Work out the finished part from the listing and answer in its coordinate system (mm). A direction names the side the tool comes from. Coordinates: 2 decimals unless noted, no trailing zeros. Write each loop counter-clockwise with the first axis right and the second up, starting at its lowest first coordinate (ties: lowest second). Pieces come first, ordered by that corner, then holes. Notation, with made-up numbers: (69, -2.75) - (87, -2.75) arc R21 cw to (87, 21.25) - close; hole circle Ø3 at (52.5, 12). An arc over 180 degrees is marked (long way). Use CSV: the item, a comma, the result in double quotes. Start each with the question number.
from build123d import *

# Parameters (mm, degrees)
F1_DEPTH = 6.35
F3_DEPTH = 52.578
F4_DEPTH = 45.974
F6_DEPTH = 4.064
F7_DEPTH = 3.81
F8_R     = 5.2545700387
F9_DEPTH = 25.4


with BuildPart() as f1:
    # F0 (on Front) → F1 (new body)
    with BuildSketch(Plane.XZ):
        Polygon((-31.1878696084, 40.077868849), (-52.4655729532, 40.077868849), (-52.4655729532, -4.226393532), (30.0219655037, -4.226393532), (30.0219655037, 19.6718552087), align=None)
    extrude(amount=F1_DEPTH)

    # F2 (on Right) → F3 (join)
    with BuildSketch(Plane.YZ):
        Polygon((-6.1209839769, -4.226393532), (-6.7039346322, 32.7909812331), (-16.3226239383, 32.7909812331), (-25.3583602607, 8.5985241458), (-25.3583602607, -4.226393532), align=None)
    extrude(amount=-F3_DEPTH)

    # F4 (cut): a face of the model
    f4_faces = [f1.faces().sort_by_distance(p)[0] for p in [
        (0, -14.7154551351, 12.274399221),
    ]]
    extrude(f4_faces, amount=-F4_DEPTH, mode=Mode.SUBTRACT)

    # F5 (on Top) → F6 (join)
    with BuildSketch(Plane.XY):
        Polygon((-46.0531152785, -6.2667215243), (-46.0531152785, -25.212623179), (-14.5737715065, -6.2667215243), align=None)
    extrude(amount=-F6_DEPTH)

    # F7 (add): a face of the model
    f7_faces = [f1.faces().sort_by_distance(p)[0] for p in [
        (-35.5533806316, -12.6216691671, 0),
    ]]
    extrude(f7_faces, amount=F7_DEPTH)

    # F8 (on face) → F9 (cut)
    with BuildSketch(Plane.XZ.offset(6.35)):
        with Locations((18.0714763701, 7.7227308384)):
            Circle(F8_R)
    extrude(amount=-F9_DEPTH, mode=Mode.SUBTRACT)


solid = f1.part
Item 1: Determine the mould class of faces 1 (the face through (-0.15, -3.13, 29.73)), 2 (the face through (-34, -14, -4.064)), 3 (the face through (22.925, -3.219, 5.71)) for opening direction X: +X half, -X half, draft (parallel to the pull), parting line (faces both ways), or undercut.
Item 2: A cutting plane is placed at D-D (z = 1). Determine the outline of the cut face in (x, y) (3 decimals), then the cut area to 3 significant figures.
Item 3: A cutting plane is placed at C-C (x = -40.5). Determine the outline of the cut face in (y, z), then the cut area to 3 significant figures.
Item 4: Straight lines are drawn through the part: probe 1 along Z at (x, y) = (-31, -11.75); probe 2 along X at (y, z) = (-9.25, 5); probe 3 along X at (y, z) = (-1.5, 15). For each, find the intervals that lie inside material, in ascending order. Write a range as [from, to].
Item 5: A cutting plane is placed at A-A (z = 26). Determine the outline of the cut face in (x, y), then the cut area to 3 significant figures.
Item 6: A cutting plane is placed at B-B (y = -17.75). Determine the outline of the cut face in (x, z), then the cut area to 3 significant figures.
Item 7: Which of the six approach directions +Z, -Z, +X, -X, +Y, -Y give full straight-line access (tool end or side, diameter ignored) to faces 4 (the face through (-34, -14, 3.81)), 5 (the face through (-18, -6, -4.226)), 6 (the face through (-49, -11, 32.791))?
Item 8: Each of these flat-tipped pins is pushed along its axis until it touches: pin 1 (5 mm diameter, centred on x = -38, z = 19.5, fed in from -Y); pin 2 (2 mm diameter, centred on x = -49, y = -10, fed in from +Z); pin 3 (1.5 mm diameter, centred on x = 14, z = 7.5, fed in from +Y); pin 4 (1.9 mm diameter, centred on y = -3.5, z = 12.5, fed in from -X). Where does it stop, or does it pass through?
Calculated:
1,face 1,"+X half"
1,face 2,"draft"
1,face 3,"undercut"
2,outline,"(-52.578, -25.358) - (-45.974, -25.358) - (-45.974, -25.165) - (-14.712, -6.35) - (30.022, -6.35) - (30.022, 0) - (-52.466, 0) - (-52.466, -6.203) - (-52.578, -6.203) - close"
2,area,"943 mm²"
3,outline,"(-21.87, -4.06) - (-6.35, -4.06) - (-6.35, -4.23) - (0, -4.23) - (0, 40.08) - (-6.35, 40.08) - (-6.35, 3.81) - (-21.87, 3.81) - close"
3,area,"404 mm²"
4,probe 1,"z = [-4.06, 3.81]"
4,probe 2,"x = [-52.58, -45.97]"
4,probe 3,"x = [-52.47, 30.02]"
5,outline,"(-52.58, -18.86) - (-45.97, -18.86) - (-45.97, -6.6) - (-52.58, -6.6) - close; (-52.47, -6.35) - (11.04, -6.35) - (11.04, 0) - (-52.47, 0) - close"
5,area,"484 mm²"
6,outline,"(-52.58, -4.23) - (-45.97, -4.23) - (-45.97, -4.06) - (-33.65, -4.06) - (-33.65, 3.81) - (-45.97, 3.81) - (-45.97, 28.97) - (-52.58, 28.97) - close"
6,area,"316 mm²"
7,face 4,"+Z, +X, -Y"
7,face 5,"-Z, +X, -X, +Y, -Y"
7,face 6,"+Z, +X, -X, -Y"
8,pin 1,"stops at y = -6.35"
8,pin 2,"stops at z = 32.79"
8,pin 3,"passes through"
8,pin 4,"stops at x = -52.47"
